```python
from build123d import *

# Parameters (mm, degrees)
F2_R     = 0.05
F3_DEPTH = 90.001


with BuildPart() as f1:
    # F0 (on Front) → F1 (revolve)
    with BuildSketch(Plane.XZ):
        with BuildLine():
            Line((10, 45), (0, 45))
            Line((0, 45), (0, 35))
            ThreePointArc((0, 35), (7.801535, 31.82176), (11.591531, 24.298391))
            ThreePointArc((11.591531, 24.298391), (12.905056, 0), (11.591531, -24.298391))
            ThreePointArc((11.591531, -24.298391), (7.801535, -31.82176), (0, -35))
            Line((0, -35), (0, -45))
            Line((0, -45), (10, -45))
            ThreePointArc((10, -45), (14.505056, 0), (10, 45))
        make_face()
    revolve(axis=Axis((0, 0, 40), (0, 0, -1)))

    # F2 (on face) → F3 (cut, through all)
    with BuildSketch(Plane.XY.offset(45)):
        Circle(F2_R)
    extrude(amount=-F3_DEPTH, mode=Mode.SUBTRACT)


solid = f1.part
```
Here's how the part is built. I have some questions about the finished solid (model axes, mm). Give positions to 0.01 mm unless a question says otherwise; leave off trailing zeros. Put each result on its own line as item: value. Start each with the question number.
Item 1: Thinking about a two-plate mould opening in Z: for faces 1 (the flat face through (-2, 0, -45)), 2 (the flat face through (2, 0, 45)), which applies, +Z half, -Z half, draft (parallel to the pull), parting line (faces both ways), or undercut?
Item 2: I need wall thicknesses on L1, parallel to Z at x = -1.5, y = 5.25; L2, parallel to Z at x = -1.5, y = -5; L3, parallel to X at y = 0, z = -31. Which ranges of each line are inside material? Lowest first, please. Write a range as from..to.
Item 3: Will these pins go through, and if not, where does the flat tip stop? pin 1 (3 mm diameter, centred on x = 7.5, z = 8.5, fed in from -Y); pin 2 (8 mm diameter, centred on x = 6.5, z = -35.5, fed in from -Y); pin 3 (3 mm diameter, centred on y = -7, z = -1.5, fed in from -X).
Values:
1. face 1: -Z half
1. face 2: +Z half
2. L1: -45..-33.51, 33.51..45
2. L2: -45..-33.64, 33.64..45
2. L3: -12.38..-8.61, 8.61..12.38
3. pin 1: y = -13.03
3. pin 2: y = -11.63
3. pin 3: x = -13.42
